Work out the finished part from the listing and answer in its coordinate system (mm). Face numbers are marked on the shaded views. A direction names the side the tool comes from. Give positions to 0.01 mm unless a question says otherwise; leave off trailing zeros. Loops run counter-clockwise (first coordinate to the right, second up) from the corner with the lowest first, then second, coordinate; pieces in that order, holes last. Notation, with made-up numbers: M 33.25,5.5 L 86.25,5.5 A33 ccw 86.25,33.5 Z; hole C 84,-1 d9. An arc over 180 degrees is marked long. Use a Markdown table: item, result.
```python
from build123d import *

# Parameters (mm, degrees)
SKETCH1_W           = 50
SKETCH1_H           = 50
BOSS_EXTRUDE1_DEPTH = 50
SKETCH3_W           = 40
SKETCH3_H           = 40
CUT_EXTRUDE1_DEPTH  = 40
SKETCH4_R           = 4
CUT_EXTRUDE2_DEPTH  = 40
SKETCH5_R           = 4
CUT_EXTRUDE3_DEPTH  = 40
SKETCH6_R           = 4
CUT_EXTRUDE4_DEPTH  = 40
FILLET1_R           = 20
FILLET2_R           = 20


with BuildPart() as part:
    # Sketch1 → Boss-Extrude1 (new body)
    with BuildSketch(Plane(origin=(0, 0, 0), x_dir=(1, 0, 0), z_dir=(0, 1, 0))):
        with Locations((25, 25)):
            Rectangle(SKETCH1_W, SKETCH1_H)
    extrude(amount=BOSS_EXTRUDE1_DEPTH)

    # Sketch3 → Cut-Extrude1 (cut)
    with BuildSketch(Plane(origin=(0, 50, 0), x_dir=(1, 0, 0), z_dir=(0, 1, 0))):
        with Locations((30, 30)):
            Rectangle(SKETCH3_W, SKETCH3_H)
    extrude(amount=-CUT_EXTRUDE1_DEPTH, mode=Mode.SUBTRACT)

    # Sketch4 → Cut-Extrude2 (cut)
    with BuildSketch(Plane(origin=(0, 10, 0), x_dir=(1, 0, 0), z_dir=(0, 1, 0))):
        with Locations(Location((40, 40, 0), (0, 0, 270))):
            Circle(SKETCH4_R)
    extrude(amount=-CUT_EXTRUDE2_DEPTH, mode=Mode.SUBTRACT)

    # Sketch5 → Cut-Extrude3 (cut)
    with BuildSketch(Plane.XY):
        with Locations((40, 40)):
            Circle(SKETCH5_R)
    extrude(amount=-CUT_EXTRUDE3_DEPTH, mode=Mode.SUBTRACT)

    # Sketch6 → Cut-Extrude4 (cut)
    with BuildSketch(Plane.ZY):
        with Locations((-40, 40)):
            Circle(SKETCH6_R)
    extrude(amount=-CUT_EXTRUDE4_DEPTH, mode=Mode.SUBTRACT)

    # Fillet1
    fillet1_edges = [part.edges().sort_by_distance(p)[0] for p in [
        (10, 30, -10),
    ]]
    fillet(fillet1_edges, radius=FILLET1_R)

    # Fillet2
    fillet2_edges = [part.edges().sort_by_distance(p)[0] for p in [
        (10, 10, -40),
        (40, 10, -10),
        (15.857864376, 10, -15.857864376),
    ]]
    fillet(fillet2_edges, radius=FILLET2_R)


solid = part.part
```
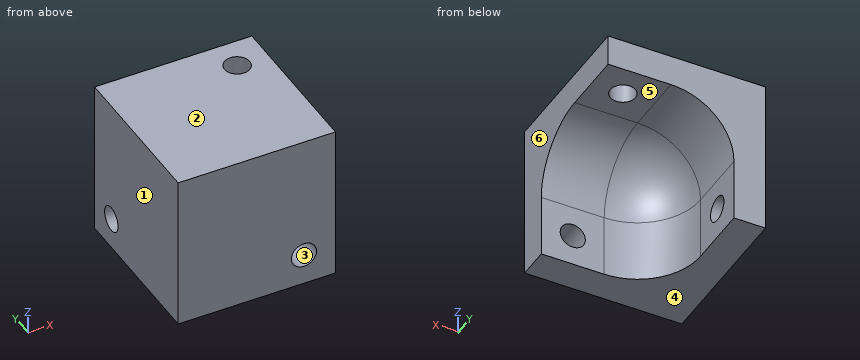
(1) A cutting plane is placed at D-D (x = 8). Write down the section's boundary in (y, z).
Entries:
| item | result |
|---|---|
| outline | M 0,-50 L 50,-50 L 50,0 L 0,0 Z; hole C 40,-40 d8 |
(2) The mould has two halves that part along Z. Classify the marked faces 1, 2, 3 and 4: released by +Z, released by -Z, zero draft, split by the parting line, or undercut.
Entries:
| item | result |
|---|---|
| face 1 | zero draft |
| face 2 | released by +Z |
| face 3 | undercut |
| face 4 | released by -Z |
(3) A cutting plane is placed at A-A (z = -40). Write down the section's boundary in (x, y), and give its area (3 significant figures).
Entries:
| item | result |
|---|---|
| outline | M 0,0 L 36,0 L 36,10 L 30,10 A20 cw 10,30 L 10,36 L 0,36 Z; M 0,44 L 10,44 L 10,50 L 0,50 Z; M 44,0 L 50,0 L 50,10 L 44,10 Z |
| area | 826 mm² |
(4) A cutting plane is placed at B-B (x = 40). Write down the section's boundary in (y, z).
Entries:
| item | result |
|---|---|
| outline | M 0,-50 L 10,-50 L 10,-44 L 0,-44 Z; M 0,-36 L 10,-36 L 10,-30 A20 cw 30,-10 L 36,-10 L 36,0 L 0,0 Z; M 44,-10 L 50,-10 L 50,0 L 44,0 Z |
(5) A cutting plane is placed at C-C (y = 32). Write down the section's boundary in (x, z), and give its area (3 significant figures).
Entries:
| item | result |
|---|---|
| outline | M 0,-50 L 10,-50 L 10,-30 A20 cw 30,-10 L 50,-10 L 50,0 L 0,0 Z |
| area | 986 mm² |
(6) Which of the six approach directions +Z, -Z, +X, -X, +Y, -Y give full straight-line access (tool end or side, diameter ignored) to the marked faces 5 and 6?
Entries:
| item | result |
|---|---|
| face 5 | -Z, +X, +Y |
| face 6 | +Z, -Z, +X, +Y, -Y |
(7) Given P1, Ø1.5, axis at y = 42, z = -19, coming from the +X side; P2, Ø6, axis at x = 39, y = 43.5, coming from the -Z side; P3, Ø1, axis at x = 36.5, z = -19, coming from the +Y side, each flat-ended and moving along its own axis, determine where each tip first touches the part or whether it passes through.
Entries:
| item | result |
|---|---|
| P1 | stops at x = 13.82 |
| P2 | stops at z = -10 |
| P3 | stops at y = 13.64 |
(8) Consider probe 1 along Y at (x, z) = (40, -6.25); probe 2 along Y at (x, z) = (47.5, -33); probe 3 along Z at (x, y) = (37.5, 30). Determine where each line is inside the solid, lowest interval first. Write a range as [from, to].
Entries:
| item | result |
|---|---|
| probe 1 | y = [0, 36], [44, 50] |
| probe 2 | y = [0, 10] |
| probe 3 | z = [-10, 0] |
